Geometry: final body of the model. Coordinates: model frame, mm. A direction names the side the tool comes from. Round coordinates to 2 decimals unless told otherwise and drop trailing zeros. Loops run counter-clockwise (first coordinate to the right, second up) from the corner with the lowest first, then second, coordinate; pieces in that order, holes last. Notation, with made-up numbers: M 17.25,21.25 L 70.25,21.25 A21 cw 70.25,56.25 Z; hole C 35,-2 d8. An arc over 180 degrees is marked long. Answer as a JSON object with one key per item and string values.
```python
from build123d import *

# Parameters (mm, degrees)
F1_DEPTH = 1422.4
F0_W     = 965.2
F0_H     = 254
F0_H_2   = 711.2
F2_DEPTH = 457.2
F8_DEPTH = 508


with BuildPart() as f1:
    # F0 (on Top) → F1 (new body)
    with BuildSketch(Plane.XY):
        Polygon((-1270, 0), (-965.2, 0), (-965.2, 711.2), (0, 711.2), (0, 1016), (-965.2, 1016), (-965.2, 1270), (-1270, 1270), (-1270, 1016), (-2235.2, 1016), (-2235.2, 711.2), (-1270, 711.2), align=None)
    extrude(amount=F1_DEPTH)

    # F0 (on Top) → F2 (join)
    with BuildSketch(Plane.XY):
        with Locations((-1752.6, 1143)):
            Rectangle(F0_W, F0_H)
        with Locations((-482.6, 1143)):
            Rectangle(F0_W, F0_H)
        with Locations((-1752.6, 355.6)):
            Rectangle(F0_W, F0_H_2)
        with Locations((-482.6, 355.6)):
            Rectangle(F0_W, F0_H_2)
    extrude(amount=F2_DEPTH)

    # F7 (on 3pt) → F8 (cut)
    with BuildSketch(Plane(origin=(0, 0, 0), x_dir=(0.8331213628, 0.4125708276, -0.3683668104), z_dir=(0.553090223, -0.6214566012, 0.5548719654))):
        Polygon((0, 0), (0, 1904.3694734573), (-1708.9967775732, 1061.0217298967), align=None)
    extrude(amount=F8_DEPTH, mode=Mode.SUBTRACT)


solid = f1.part
```
1) Pull-direction query (Z, two-part tool) for faces 6 (the face through (-1759, 1145, 457.2)), 7 (the face through (-1115.42, 274.41, 1421.66)), 8 (the face through (0, 767, 308)); classes: +Z half, -Z half, draft (parallel to the pull), parting line (faces both ways), or undercut.
Geometry results:
{"face 6": "+Z half", "face 7": "undercut", "face 8": "draft"}
2) Cut plane B-B on x = -1764.5. Return the cut outline in (y, z).
Geometry results:
{"outline": "M 0,0 L 1270,0 L 1270,457.2 L 1016,457.2 L 1016,1422.4 L 711.2,1422.4 L 711.2,457.2 L 0,457.2 Z"}
3) Cut plane C-C on y = 550. Return the cut outline in (x, z), and give its area (3 significant figures).
Geometry results:
{"outline": "M -2235.2,0 L 0,0 L 0,457.2 L -965.2,457.2 L -965.2,1422.4 L -1270,1422.4 L -1270,457.2 L -2235.2,457.2 Z", "area": "1,320,000 mm2"}
4) Cut plane D-D on x = -357.5. Return the cut outline in (y, z), and give its area (3 significant figures).
Geometry results:
{"outline": "M 0,0 L 1270,0 L 1270,457.2 L 1016,457.2 L 1016,1422.4 L 946.77,1422.4 L 950.27,1420.65 L 711.2,1152.9 L 711.2,457.2 L 90.04,457.2 L 0.4,356.79 L 0,357.5 Z", "area": "838,000 mm2"}
5) Cut plane A-A on z = 659. Return the cut outline in (x, y).
Geometry results:
{"outline": "M -2235.2,711.2 L -1270,711.2 L -1270,0 L -965.2,0 L -965.2,711.2 L 0,711.2 L 0,1016 L -965.2,1016 L -965.2,1270 L -1270,1270 L -1270,1016 L -2235.2,1016 Z"}
6) Set-up query: faces 1 (the face through (-450.517, 865.761, 1421.557)), 2 (the face through (-965.2, 1141, 933)), 3 (the face through (-1759, 361, 457.2)), 4 (the face through (-597, 711.2, 826)), 5 (the face through (-1270, 1145, 933)). Return all of +Z, -Z, +X, -X, +Y, -Y with unobstructed straight access to the full face (end or side cutting, diameter ignored); none if empty.
Geometry results:
{"face 1": "+X, -Y", "face 2": "+Z, +X, +Y", "face 3": "+Z, -X, -Y", "face 4": "+Z, +X, -Y", "face 5": "+Z, -X, +Y"}
7) First-contact query: pin 1 (6 mm diameter, centred on x = -794.5, y = 228.5, fed in from +Z). Flat tip, straight axial feed; report the tip coordinate or a pass-through.
Geometry results:
{"pin 1": "z = 457.2"}
8) Line query: probe 1 along Z at (x, y) = (-778, 1177); probe 2 along Y at (x, z) = (-1605.5, 1002); probe 3 along X at (y, z) = (421.5, 895.5). Output: solid intervals per line, ascending.
Geometry results:
{"probe 1": "0 to 457.2", "probe 2": "711.2 to 1016", "probe 3": "-1270 to -965.2"}
